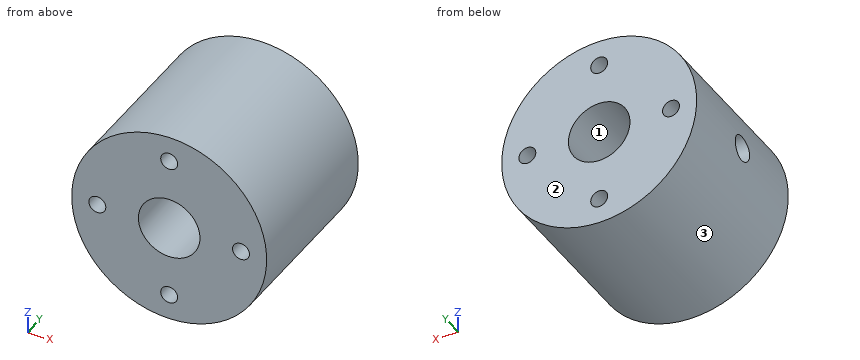
from build123d import *

# Parameters (mm, degrees)
SKETCH_1_R             = 19
SKETCH_1_R_2           = 6
EXTRUDE_1_DEPTH        = 32
SKETCH_2_R             = 2.5
CUT_EXTRUDE_1_DEPTH    = 42.785164832
HOLE_WIZARD_M4_1_D     = 3.3
HOLE_WIZARD_M4_1_DEPTH = 10.1
HOLE_WIZARD_M4_1_TIP   = 0.991420021
HOLE_WIZARD_M4_2_D     = 3.3
HOLE_WIZARD_M4_2_DEPTH = 10.1
HOLE_WIZARD_M4_2_TIP   = 0.991420021


with BuildPart() as part:
    # 草图1 → 凸台-拉伸1 (new body)
    with BuildSketch(Plane(origin=(0, 0, 0), x_dir=(1, 0, 0), z_dir=(0, 1, 0))):
        with Locations(Location((0, 0, 0), (0, 0, 270))):
            Circle(SKETCH_1_R)
        with Locations(Location((0, 0, 0), (0, 0, 270))):
            Circle(SKETCH_1_R_2, mode=Mode.SUBTRACT)
    extrude(amount=EXTRUDE_1_DEPTH)

    # 草图2 → 切除-拉伸1 (cut, through all)
    with BuildSketch(Plane(origin=(0, 0, 0), x_dir=(0, 0, -1), z_dir=(1, 0, 0))):
        with Locations((0, 16)):
            Circle(SKETCH_2_R)
    extrude(amount=-CUT_EXTRUDE_1_DEPTH, mode=Mode.SUBTRACT)

    # M4 螺纹孔1
    with Locations(Plane(origin=(0, 32, 0), x_dir=(-1, 0, 0), z_dir=(0, 1, 0))):
        with Locations((14, 0), (0, 14), (-14, 0), (0, -14)):
            Hole(HOLE_WIZARD_M4_1_D / 2, depth=HOLE_WIZARD_M4_1_DEPTH)
            with Locations((0, 0, -(HOLE_WIZARD_M4_1_DEPTH + HOLE_WIZARD_M4_1_TIP / 2))):  # 118° drill point
                Cone(0, HOLE_WIZARD_M4_1_D / 2, HOLE_WIZARD_M4_1_TIP, mode=Mode.SUBTRACT)

    # M4 螺纹孔2
    with Locations(Plane.XZ):
        with Locations((0, 14), (-14, 0), (0, -14), (14, 0)):
            Hole(HOLE_WIZARD_M4_2_D / 2, depth=HOLE_WIZARD_M4_2_DEPTH)
            with Locations((0, 0, -(HOLE_WIZARD_M4_2_DEPTH + HOLE_WIZARD_M4_2_TIP / 2))):  # 118° drill point
                Cone(0, HOLE_WIZARD_M4_2_D / 2, HOLE_WIZARD_M4_2_TIP, mode=Mode.SUBTRACT)


solid = part.part
Read the model definition and answer for the solid it produces. Units are mm, in the model's axes. Face numbers are marked on the shaded views. Round coordinates to 2 decimals unless told otherwise and drop trailing zeros. Write each loop counter-clockwise with the first axis right and the second up, starting at its lowest first coordinate (ties: lowest second). Pieces come first, ordered by that corner, then holes. Notation, with made-up numbers: (5.25, -32.5) - (63.25, -32.5) arc R25 ccw to (63.25, -18.5) - close; hole circle Ø9 at (27, 56.25). An arc over 180 degrees is marked (long way). One line per question, with ' | ' between items. Start each with the question number.
1. For a pull along X with two mould halves and no side action, classify the marked faces 1, 2 and 3 as +X half, -X half, draft (parallel to the pull), parting line (faces both ways), or undercut.
2. Each of these flat-tipped pins is pushed along its axis until it touches: pin 1 (3 mm diameter, centred on y = 16, z = 0, fed in from +X); pin 2 (2 mm diameter, centred on x = -14, z = 0, fed in from -Y); pin 3 (6 mm diameter, centred on y = 28, z = 5, fed in from -X). Where does it stop, or does it pass through?
3. Section C-C (y = 20) is taken. Determine the outline of the cut face in (x, z).
4. Find the intervals of material crossed by probe 1 along X at (y, z) = (3.25, -14); probe 2 along Z at (x, y) = (3.5, 8.5), in increasing order. Write a range as [from, to].
5. Section D-D (y = 16) is taken. Determine the outline of the cut face in (x, z).
6. Section A-A (y = 28.5) is taken. Determine the outline of the cut face in (x, z), and give its area (3 significant figures).
7. Section B-B (x = -4.5) is taken. Determine the outline of the cut face in (y, z), and give its area (3 significant figures).
Filled in:
1) face 1: undercut | face 2: draft | face 3: parting line
2) pin 1: x = 19 | pin 2: y = 10.49 | pin 3: x = -18.89
3) outline: circle Ø38 at (0, 0); hole circle Ø12 at (0, 0)
4) probe 1: [-12.85, -1.65], [1.65, 12.85] | probe 2: [-18.67, -4.87], [4.87, 18.67]
5) outline: (-18.83, -2.5) arc R19 ccw (long way) to (-18.83, 2.5) - (-5.45, 2.5) arc R6 cw (long way) to (-5.45, -2.5) - close
6) outline: circle Ø38 at (0, 0); hole circle Ø3.3 at (-14, 0); hole circle Ø12 at (0, 0); hole circle Ø3.3 at (0, -14); hole circle Ø3.3 at (0, 14); hole circle Ø3.3 at (14, 0) | area: 987 mm²
7) outline: (0, -18.46) - (32, -18.46) - (32, -3.97) - (0, -3.97) - close; (0, 3.97) - (32, 3.97) - (32, 18.46) - (0, 18.46) - close | area: 927 mm²
